Geometry check sheet. Reference: the model listing, model coordinates, mm. Face numbers are marked on the shaded views. A direction names the side the tool comes from. Coordinates: 2 decimals unless noted, no trailing zeros. Write each loop counter-clockwise with the first axis right and the second up, starting at its lowest first coordinate (ties: lowest second). Pieces come first, ordered by that corner, then holes. Notation, with made-up numbers: M 84.5,19.5 L 88.5,19.5 A15 cw 88.5,41.5 Z; hole C 34,45 d3. An arc over 180 degrees is marked long. Put each result on its own line as item: value. Start each with the question number.
1) Set-up check for the marked faces 1, 2, 3 and 4: record each of +Z, -Z, +X, -X, +Y, -Y from which the full face is reachable in a straight line by a thin tool's end or side.
2) Cross-section at A-A on z = 2.75. Record the cut outline in (x, y), plus the area to 3 significant figures.
3) Cross-section at C-C on z = 10. Record the cut outline in (x, y), plus the area to 3 significant figures.
4) Gauge pin test, flat ends, axial feed: pin 1 (1.5 mm diameter, centred on x = 9, y = 1, fed in from -Z); pin 2 (5 mm diameter, centred on y = 1, z = 5.5, fed in from -X); pin 3 (0.7 mm diameter, centred on x = 7, y = 1.5, fed in from +Z). Record the tip position at first contact, or that the pin passes through.
5) Mould release check, pull along X, two halves, no side actions. Record for the marked faces 5, 6 and 7: released by +X, released by -X, zero draft, split by the parting line, or undercut.
6) Scan lines: line 1 along X through (y, z) = (-2.75, 10.25); line 2 along Y through (x, z) = (-8.25, 9.25); line 3 along Z through (x, y) = (1.5, -1.75). Record each from-to range of solid material in increasing order.
7) Cross-section at B-B on y = 1.75. Record the cut outline in (x, z), plus the area to 3 significant figures.
8) Cross-section at D-D on y = -2.75. Record the cut outline in (x, z), plus the area to 3 significant figures.
from build123d import *

# Parameters (mm, degrees)
SKETCH_1_W          = 12
SKETCH_1_H          = 12
EXTRUDE_1_DEPTH     = 1.35
SKETCH_2_W          = 11.32
SKETCH_2_H          = 12
EXTRUDE_2_DEPTH     = 1.35
EXTRUDE_3_DEPTH     = 2.7
CUT_EXTRUDE_1_DEPTH = 3
CHAMFER_1_SIZE      = 1
FILLET_1_R          = 1


with BuildPart() as part:
    # 草图1 → 凸台-拉伸1 (new body)
    with BuildSketch(Plane.XY):
        Rectangle(SKETCH_1_W, SKETCH_1_H)
    extrude(amount=EXTRUDE_1_DEPTH)

    # 草图2 → 凸台-拉伸2 (add)
    with BuildSketch(Plane.ZY.offset(6)):
        with Locations((5.66, 0)):
            Rectangle(SKETCH_2_W, SKETCH_2_H)
    extrude_2 = extrude(amount=EXTRUDE_2_DEPTH)

    # 草图3 → 凸台-拉伸3 (add)
    with BuildSketch(Plane.XY.offset(11.32)):
        with BuildLine():
            Line((-7.35, 6), (-8.25, 6))
            ThreePointArc((-8.25, 6), (-12.5, 1.75), (-8.25, -2.5))
            Line((-8.25, -2.5), (-7.35, -2.5))
            Line((-7.35, -2.5), (-7.35, 6))
        make_face()
    extrude_3 = extrude(amount=-EXTRUDE_3_DEPTH)

    # 草图4 → 切除-拉伸1 (cut)
    with BuildSketch(Plane.XY.offset(11.32)):
        with BuildLine():
            Line((-6, 3.05), (-8.7, 3.05))
            ThreePointArc((-8.7, 3.05), (-10, 1.75), (-8.7, 0.45))
            Line((-8.7, 0.45), (-6, 0.45))
            Line((-6, 0.45), (-6, 3.05))
        make_face()
    cut_extrude_1 = extrude(amount=-CUT_EXTRUDE_1_DEPTH, mode=Mode.SUBTRACT)

    # 镜向1: 凸台-拉伸2, 凸台-拉伸3, 切除-拉伸1 across plane
    add(extrude_2.mirror(Plane(origin=(0, 0, 0), x_dir=(0, 0, 1), z_dir=(1, 0, 0))))
    add(extrude_3.mirror(Plane(origin=(0, 0, 0), x_dir=(0, 0, 1), z_dir=(1, 0, 0))))
    add(cut_extrude_1.mirror(Plane(origin=(0, 0, 0), x_dir=(0, 0, 1), z_dir=(1, 0, 0))), mode=Mode.SUBTRACT)

    # 倒角1
    chamfer_1_edges = [part.edges().sort_by_distance(p)[0] for p in [
        (-6, 0, 1.35),
        (6, 0, 1.35),
    ]]
    chamfer(chamfer_1_edges, length=CHAMFER_1_SIZE)

    # 圆角1
    fillet_1_edges = [part.edges().sort_by_distance(p)[0] for p in [
        (-7.35, 0, 0),
        (7.35, 0, 0),
    ]]
    fillet(fillet_1_edges, radius=FILLET_1_R)


solid = part.part
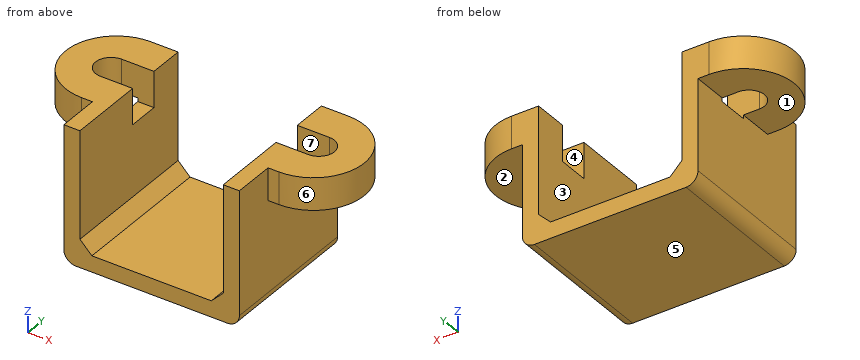
Answer key:
1. face 1: -Z, -X, +Y, -Y
1. face 2: -Z, +X, +Y, -Y
1. face 3: +Z, +Y, -Y
1. face 4: +Z
2. outline: M -7.35,-6 L -6,-6 L -6,6 L -7.35,6 Z; M 6,-6 L 7.35,-6 L 7.35,6 L 6,6 Z
2. area: 32.4 mm²
3. outline: M -8.7,0.45 A1.3 cw -8.7,3.05 L -6,3.05 L -6,6 L -8.25,6 A4.25 ccw -8.25,-2.5 L -7.35,-2.5 L -7.35,-6 L -6,-6 L -6,0.45 Z; M 6,-6 L 7.35,-6 L 7.35,-2.5 L 8.25,-2.5 A4.25 ccw 8.25,6 L 6,6 L 6,3.05 L 8.7,3.05 A1.3 cw 8.7,0.45 L 6,0.45 Z
3. area: 85.1 mm²
4. pin 1: stops at z = 8.62
4. pin 2: stops at x = -7.35
4. pin 3: stops at z = 8.32
5. face 5: zero draft
5. face 6: released by +X
5. face 7: undercut
6. line 1: x = -7.35 to -6, 6 to 7.35
6. line 2: y = -2.5 to 0.45, 3.05 to 6
6. line 3: z = 0 to 1.35
7. outline: M -12.5,8.62 L -10,8.62 L -10,11.32 L -12.5,11.32 Z; M -7.35,1 A1 ccw -6.35,0 L 6.35,0 A1 ccw 7.35,1 L 7.35,8.32 L 6,8.32 L 6,2.35 L 5,1.35 L -5,1.35 L -6,2.35 L -6,8.32 L -7.35,8.32 Z; M 10,8.62 L 12.5,8.62 L 12.5,11.32 L 10,11.32 Z
7. area: 52.7 mm²
8. outline: M -7.35,1 A1 ccw -6.35,0 L 6.35,0 A1 ccw 7.35,1 L 7.35,11.32 L 6,11.32 L 6,2.35 L 5,1.35 L -5,1.35 L -6,2.35 L -6,11.32 L -7.35,11.32 Z
8. area: 47.3 mm²
